Source: CAD feature listing. Evaluate the final solid. Frame: model axes, mm. Face numbers are marked on the shaded views. A direction names the side the tool comes from. Round coordinates to 2 decimals unless told otherwise and drop trailing zeros. Write each loop counter-clockwise with the first axis right and the second up, starting at its lowest first coordinate (ties: lowest second). Pieces come first, ordered by that corner, then holes. Notation, with made-up numbers: M 11.5,-17.5 L 55.5,-17.5 A20 cw 55.5,0.5 Z; hole C 84,-22 d1. An arc over 180 degrees is marked long. Put each result on its own line as item: value. Start each with the question number.
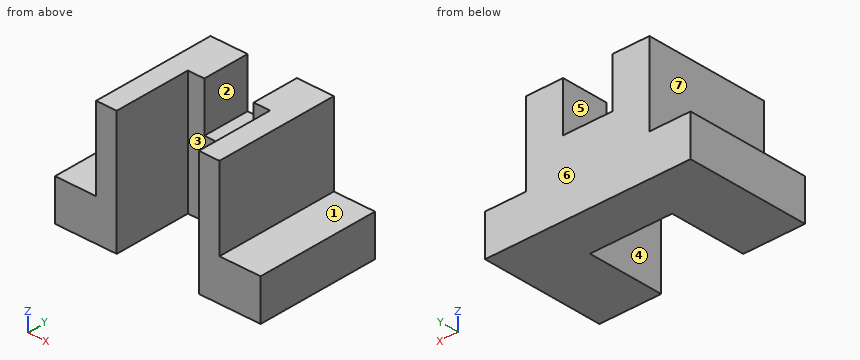
```python
from build123d import *

# Parameters (mm, degrees)
F1_DEPTH = 45
F2_W     = 30
F2_H     = 28
F3_DEPTH = 45.001


with BuildPart() as f1:
    # F0 (on Front) → F1 (new body)
    with BuildSketch(Plane.XZ):
        Polygon((-37.5, 0), (0, 0), (37.5, 0), (37.5, 15), (22.5, 15), (22.5, 45), (9, 45), (9, 27), (-9, 27), (-9, 45), (-22.5, 45), (-22.5, 15), (-37.5, 15), align=None)
    extrude(amount=F1_DEPTH)

    # F2 (on face) → F3 (cut, through all)
    with BuildSketch(Plane.XY.offset(45)):
        with Locations((0, -31)):
            Rectangle(F2_W, F2_H)
    extrude(amount=-F3_DEPTH, mode=Mode.SUBTRACT)


solid = f1.part
```
(1) Section query C-C (y = -12). Return loops of the section in (x, z), and give its area (3 significant figures).
(2) Section query D-D (z = 24.5). Return loops of the section in (x, y).
(3) Ray query, line 1 along X through (y, z) = (-9.5, 37.5); line 2 along X through (y, z) = (-43, 19.5); line 3 along Y through (x, z) = (-14, 43.5). Return the intervals inside material, ascending.
(4) Access query for the marked faces 1, 2 and 3. Directions: +Z, -Z, +X, -X, +Y, -Y. A direction counts if a zero-diameter tool reaches every point of the face in a straight line with its end or side. Return the directions, or none.
(5) Pull-direction query (X, two-part tool) for the marked faces 4, 5, 6 and 7; classes: +X half, -X half, draft (parallel to the pull), parting line (faces both ways), or undercut.
(6) Section query A-A (z = 32). Return loops of the section in (x, y), and give its area (3 significant figures).
(7) Contact query for flat-ended pins moving along their axis: P1, Ø15, axis at y = -25, z = 28, coming from the -X side; P2, Ø15, axis at y = -30, z = 26, coming from the +X side; P3, Ø12, axis at x = 33, y = -18, coming from the +Z side. Output: stop coordinate, or through.
(8) Section query B-B (y = -18). Return loops of the section in (x, z), and give its area (4 significant figures).
Entries:
1. outline: M -37.5,0 L 37.5,0 L 37.5,15 L 22.5,15 L 22.5,45 L 9,45 L 9,27 L -9,27 L -9,45 L -22.5,45 L -22.5,15 L -37.5,15 Z
1. area: 2,150 mm2
2. outline: M -22.5,-45 L -15,-45 L -15,-17 L 15,-17 L 15,-45 L 22.5,-45 L 22.5,0 L -22.5,0 Z
3. line 1: -22.5 to -9, 9 to 22.5
3. line 2: -22.5 to -15, 15 to 22.5
3. line 3: -17 to 0
4. face 1: +Z, +X, +Y, -Y
4. face 2: +Z, +Y, -Y
4. face 3: +Z, -Z, -Y
5. face 4: undercut
5. face 5: undercut
5. face 6: draft
5. face 7: -X half
6. outline: M -22.5,-45 L -15,-45 L -15,-17 L -9,-17 L -9,0 L -22.5,0 Z; M 9,-17 L 15,-17 L 15,-45 L 22.5,-45 L 22.5,0 L 9,0 Z
6. area: 879 mm2
7. P1: x = -22.5
7. P2: x = 22.5
7. P3: z = 15
8. outline: M -37.5,0 L -15,0 L -15,45 L -22.5,45 L -22.5,15 L -37.5,15 Z; M 15,0 L 37.5,0 L 37.5,15 L 22.5,15 L 22.5,45 L 15,45 Z
8. area: 1,125 mm2
